Input: part model. Units: mm. Frame: model coordinates. A direction names the side the tool comes from. Give positions to 0.01 mm unless a question says otherwise; leave off trailing zeros. Loops run counter-clockwise (first coordinate to the right, second up) from the corner with the lowest first, then second, coordinate; pieces in that order, holes last. Notation, with made-up numbers: (17.25, 17) - (34.25, 17) arc R23 ccw to (34.25, 50) - close; hole circle Ø11 at (72, 48.25). An arc over 180 degrees is marked (long way). Answer as a JSON object with one key per item and string values.
from build123d import *

# Parameters (mm, degrees)
SKETCH7_W               = 200
SKETCH7_H               = 160
BOSS_EXTRUDE5_DEPTH     = 5
SKETCH8_R               = 1.5
CUT_EXTRUDE2_DEPTH      = 129.16005618
MIRROR5_COPY_1_SKETCH_R = 1.5
MIRROR5_COPY_1_DEPTH    = 129.16005618
SKETCH11_R              = 1.5
CUT_EXTRUDE8_DEPTH      = 129.16005618
SKETCH15_R              = 1.5
CUT_EXTRUDE13_DEPTH     = 129.16005618
SKETCH17_R              = 1.5
CUT_EXTRUDE16_DEPTH     = 129.16005618
SKETCH18_R              = 1.5
CUT_EXTRUDE20_DEPTH     = 129.16005618
FILLET1_R               = 1
SKETCH19_W              = 15.093823339
SKETCH19_H              = 31.414282074
CUT_EXTRUDE21_DEPTH     = 129.16005618


with BuildPart() as part:
    # Sketch7 → Boss-Extrude5 (new body)
    with BuildSketch(Plane(origin=(0, 0, 0), x_dir=(1, 0, 0), z_dir=(0, 1, 0))):
        Rectangle(SKETCH7_W, SKETCH7_H)
    extrude(amount=BOSS_EXTRUDE5_DEPTH)

    # Sketch8 → Cut-Extrude2 (cut, through all)
    with BuildSketch(Plane(origin=(0, 0, 0), x_dir=(-1, 0, 0), z_dir=(0, -1, 0))):
        with Locations(Location((92.5, -72.5, 0), (0, 0, 90))):
            Circle(SKETCH8_R)
    cut_extrude2 = extrude(amount=-CUT_EXTRUDE2_DEPTH, mode=Mode.SUBTRACT)

    # Mirror4: Cut-Extrude2 across plane
    add(cut_extrude2.mirror(Plane.XY), mode=Mode.SUBTRACT)

    # Mirror5: Cut-Extrude2 across plane
    add(cut_extrude2.mirror(Plane(origin=(0, 0, 0), x_dir=(0, 0, 1), z_dir=(1, 0, 0))), mode=Mode.SUBTRACT)

    # Mirror5 copy 1 sketch → Mirror5 copy 1 (cut, through all)
    with BuildSketch(Plane.XZ):
        with Locations(Location((92.5, -72.5, 0), (0, 0, 90))):
            Circle(MIRROR5_COPY_1_SKETCH_R)
    extrude(amount=-MIRROR5_COPY_1_DEPTH, mode=Mode.SUBTRACT)

    # Sketch11 → Cut-Extrude8 (cut, through all)
    with BuildSketch(Plane(origin=(0, 0, 0), x_dir=(-1, 0, 0), z_dir=(0, -1, 0))):
        with Locations(Location((36.83, -58.98, 0), (0, 0, 90))):
            Circle(SKETCH11_R)
        with Locations(Location((36.83, 35, 0), (0, 0, 90))):
            Circle(SKETCH11_R)
        with Locations(Location((-36.83, -58.98, 0), (0, 0, 270))):
            Circle(SKETCH11_R)
        with Locations(Location((-36.83, 35, 0), (0, 0, 270))):
            Circle(SKETCH11_R)
    extrude(amount=-CUT_EXTRUDE8_DEPTH, mode=Mode.SUBTRACT)

    # Sketch15 → Cut-Extrude13 (cut, through all)
    with BuildSketch(Plane(origin=(0, 0, 0), x_dir=(-1, 0, 0), z_dir=(0, -1, 0))):
        with Locations(Location((70, -55, 0), (0, 0, 90))):
            Circle(SKETCH15_R)
        with Locations(Location((70, 55, 0), (0, 0, 270))):
            Circle(SKETCH15_R)
        with Locations(Location((-70, 55, 0), (0, 0, 90))):
            Circle(SKETCH15_R)
        with Locations(Location((-70, -55, 0), (0, 0, 270))):
            Circle(SKETCH15_R)
    extrude(amount=-CUT_EXTRUDE13_DEPTH, mode=Mode.SUBTRACT)

    # Sketch17 → Cut-Extrude16 (cut, through all)
    with BuildSketch(Plane(origin=(0, 0, 0), x_dir=(-1, 0, 0), z_dir=(0, -1, 0))):
        with Locations(Location((75, 0, 0), (0, 0, 90))):
            Circle(SKETCH17_R)
        with Locations(Location((-75, 0, 0), (0, 0, 270))):
            Circle(SKETCH17_R)
    extrude(amount=-CUT_EXTRUDE16_DEPTH, mode=Mode.SUBTRACT)

    # Sketch18 → Cut-Extrude20 (cut, through all)
    with BuildSketch(Plane(origin=(0, 0, 0), x_dir=(-1, 0, 0), z_dir=(0, -1, 0))):
        with Locations(Location((0, 62, 0), (0, 0, 90))):
            Circle(SKETCH18_R)
        with Locations(Location((-16, 62, 0), (0, 0, 90))):
            Circle(SKETCH18_R)
    cut_extrude20 = extrude(amount=-CUT_EXTRUDE20_DEPTH, mode=Mode.SUBTRACT)

    # Mirror12: Cut-Extrude20 across plane
    add(cut_extrude20.mirror(Plane(origin=(0, 0, 0), x_dir=(0, 0, 1), z_dir=(1, 0, 0))), mode=Mode.SUBTRACT)

    # Fillet1
    fillet1_edges = [part.edges().sort_by_distance(p)[0] for p in [
        (-100, 5, 0),
        (0, 5, 80),
        (100, 5, 0),
        (0, 0, 80),
        (-100, 0, 0),
        (0, 0, -80),
        (100, 0, 0),
        (100, 2.5, 80),
        (-100, 2.5, 80),
        (-100, 2.5, -80),
        (100, 2.5, -80),
        (0, 5, -80),
    ]]
    fillet(fillet1_edges, radius=FILLET1_R)

    # Sketch19 → Cut-Extrude21 (cut, through all)
    with BuildSketch(Plane(origin=(0, 5, 0), x_dir=(1, 0, 0), z_dir=(0, 1, 0))):
        with Locations((-54.908539981, 0)):
            Rectangle(SKETCH19_W, SKETCH19_H)
        with Locations((54.908539981, 0)):
            Rectangle(SKETCH19_W, SKETCH19_H)
    extrude(amount=-CUT_EXTRUDE21_DEPTH, mode=Mode.SUBTRACT)


solid = part.part
Item 1: Access query for faces 3 (the face through (-1, 5, -1)), 4 (the face through (55, 3, -15.707)). Directions: +Z, -Z, +X, -X, +Y, -Y. A direction counts if a zero-diameter tool reaches every point of the face in a straight line with its end or side. Return the directions, or none.
Geometry check:
{"face 3": "+Z, -Z, +X, -X, +Y", "face 4": "+Y, -Y"}
Item 2: Cut plane B-B (y = 1.9). Give the number of separate pieces and of enclosed holes in the cut face, then the cut area to 3 significant figures.
Geometry check:
{"separate pieces": "1", "enclosed holes": "19", "area": "30,900 mm2"}
Item 3: Mould query, pull axis Z, two halves, no side actions, for faces 1 (the face through (-1, 0, -1)), 2 (the face through (-55, 3, 15.707)). Classes: released by +Z, released by -Z, zero draft, split by the parting line, or undercut.
Geometry check:
{"face 1": "zero draft", "face 2": "undercut"}
Item 4: Material intervals for line 1 (Z direction, x = -70, y = 2.6); line 2 (X direction, y = 1.5, z = -72.5); line 3 (Z direction, x = -16, y = 2.5), sorted ascending. Write a range as [from, to].
Geometry check:
{"line 1": "z = [-80, -56.5], [-53.5, 53.5], [56.5, 80]", "line 2": "x = [-100, -94], [-91, 91], [94, 100]", "line 3": "z = [-80, -63.5], [-60.5, 80]"}
Item 5: Cut plane A-A (x = -58.5). Return loops of the section in (y, z).
Geometry check:
{"outline": "(0, -79) arc R1 ccw to (1, -80) - (4, -80) arc R1 ccw to (5, -79) - (5, -15.71) - (0, -15.71) - close; (0, 15.71) - (5, 15.71) - (5, 79) arc R1 ccw to (4, 80) - (1, 80) arc R1 ccw to (0, 79) - close"}
